from build123d import *

# Parameters (mm, degrees)
F0_W     = 80
F0_H     = 20
F0_W_2   = 5
F0_H_2   = 5
F1_DEPTH = 5
F2_R     = 5


# Not quite as in the source:
# - a feature names something its author has since deleted; it is built from what else it names


with BuildPart() as f1:
    # F0 (on Right) → F1 (new body)
    with BuildSketch(Plane.YZ):
        with Locations((75, 42)):
            Rectangle(F0_W, F0_H)
        with BuildLine():
            ThreePointArc((107, 48), (110.5355339059, 46.5355339059), (112, 43))
            ThreePointArc((112, 43), (110.5355339059, 39.4644660941), (107, 38))
            Line((107, 38), (57, 38))
            ThreePointArc((57, 38), (52, 43), (57, 48))
            Line((57, 48), (107, 48))
        make_face(mode=Mode.SUBTRACT)
        Polygon((35, 52), (-35, 52), (-35, 0), (-30, 0), (-30, 27.9), (19, 27.9), (19, 0), (24, 0), (35, 0), (35, 32), align=None)
        with Locations((21.5, -2.5)):
            Rectangle(F0_W_2, F0_H_2)
        with Locations((-32.5, -2.5)):
            Rectangle(F0_W_2, F0_H_2)
    extrude(amount=F1_DEPTH)

    # F2
    f2_edges = [f1.edges().sort_by_distance(p)[0] for p in [
        (2.5, 115, 52),
        (2.5, 115, 32),
    ]]
    fillet(f2_edges, radius=F2_R)


solid = f1.part
Here's how the part is built. I have some questions about the finished solid (model axes, mm). A direction names the side the tool comes from. Round coordinates to 2 decimals unless told otherwise and drop trailing zeros. Loops run counter-clockwise (first coordinate to the right, second up) from the corner with the lowest first, then second, coordinate; pieces in that order, holes last. Notation, with made-up numbers: (55.5, -23.75) - (59.5, -23.75) arc R25 ccw to (59.5, 12.25) - close; hole circle Ø11 at (4.5, 3). An arc over 180 degrees is marked (long way). One line per question, with ' | ' between items. Start each with the question number.
Q1. For faces 1 (the cylindrical face through (2, 52, 43)), 2 (the flat face through (2, 72, 32)), 3 (the flat face through (2, -6, 27.9)), 4 (the flat face through (2, -33, -5)), which set-ups out of +Z, -Z, +X, -X, +Y, -Y let a thin tool reach every point of the face, with its end or its side?
Q2. I want a section at B-B (y = 105). Write out the boundary of the cut face in (x, z), then the cut area to 3 significant figures.
Q3. Please list where these lines run through material, in increasing order: line 1 (Z direction, x = 3.85, y = 66); line 2 (Y direction, x = 3, z = 27); line 3 (Y direction, x = 0.55, z = -2). Write a range as [from, to].
Q4. I want a section at A-A (z = 2.5). Write out the boundary of the cut face in (x, y), then the cut area to 3 significant figures.
Q5. We'd pull the mould along Y, two halves only. Please class faces 5 (the flat face through (2, 115, 42)), 6 (the flat face through (2, 82, 38)), 7 (the flat face through (2, 39, 52)), 8 (the flat face through (2, -30, 11)): +Y half, -Y half, draft (parallel to the pull), parting line (faces both ways), or undercut.
Q6. I want a section at D-D (y = 39). Write out the boundary of the cut face in (x, z).
Q7. I want a section at C-C (x = 2.2). Write out the boundary of the cut face in (y, z).
Q8. Will these pins go through, and if not, where does the flat tip stop? pin 1 (1 mm diameter, centred on x = 2, z = 2, fed in from +Y); pin 2 (1.5 mm diameter, centred on x = 3.5, y = 93, fed in from -Z); pin 3 (1.5 mm diameter, centred on x = 3.5, y = 31.5, fed in from -Z).
Response values:
1) face 1: +X, -X | face 2: -Z, +X, -X, +Y | face 3: -Z, +X, -X | face 4: -Z, +X, -X, +Y, -Y
2) outline: (0, 32) - (5, 32) - (5, 38) - (0, 38) - close; (0, 48) - (5, 48) - (5, 52) - (0, 52) - close | area: 50.0 mm²
3) line 1: z = [32, 38], [48, 52] | line 2: y = [-35, -30], [19, 35] | line 3: y = [-35, -30], [19, 24]
4) outline: (0, -35) - (5, -35) - (5, -30) - (0, -30) - close; (0, 19) - (5, 19) - (5, 35) - (0, 35) - close | area: 105 mm²
5) face 5: +Y half | face 6: undercut | face 7: draft | face 8: undercut
6) outline: (0, 32) - (5, 32) - (5, 52) - (0, 52) - close
7) outline: (-35, -5) - (-30, -5) - (-30, 27.9) - (19, 27.9) - (19, -5) - (24, -5) - (24, 0) - (35, 0) - (35, 32) - (110, 32) arc R5 ccw to (115, 37) - (115, 47) arc R5 ccw to (110, 52) - (-35, 52) - close; hole (57, 38) - (107, 38) arc R5 ccw to (107, 48) - (57, 48) arc R5 ccw to start
8) pin 1: stops at y = 35 | pin 2: stops at z = 32 | pin 3: stops at z = 0
